Autodesk Inventor part; units mm, degrees
ref_plane "YZ Plane" through (0, 0, 0) normal (1, 0, 0) x (0, 1, 0)
ref_plane "XZ Plane" through (0, 0, 0) normal (0, 1, 0) x (-1, 0, 0)
ref_plane "XY Plane" through (0, 0, 0) normal (0, 0, 1) x (1, 0, 0)
sketch "Sketch1" plane through (0, 0, 0) normal (0, 0, 1) x (1, 0, 0)
  line L0 (2.2943, 2.9258) -> (2.2943, -105.0242)
  line L1 (2.2943, 2.9258) -> (90.7218, 64.8434)
  line L2 (90.7218, 64.8434) -> (27.6787, -10.2885)
  line L3 (2.2943, -105.0242) -> (27.6787, -10.2885)
  point P0 (0, 0)
  dimension "d0" = 107.95
  dimension "d1" = 107.95
extrude "Extrusion1" add sketch "Sketch1" along normal blind 3.175
sketch "Sketch2" plane through (0, 0, 0) normal (0, 0, -1) x (-1, 0, 0)
  line L0 (-2.2943, 2.9258) -> (-2.2943, -105.0242)
  line L1 (-2.2943, -51.0492) -> (-5.4693, -51.0492)
  line L2 (-5.4693, -51.0492) -> (-5.4693, -12.9492)
  line L3 (-5.4693, -12.9492) -> (-2.2943, -12.9492)
  point P0 (0, 0)
  dimension "d8" = 3.175
  dimension "d9" = 38.1
extrude "Extrusion2" add sketch "Sketch2" along normal blind 79.2734
sketch "Sketch3" plane through (2.2943, -105.0242, 3.175) normal (-1, 0, 0) x (0, 0, 1)
  line L0 (-82.4484, 92.075) -> (-63.3984, 92.075)
  line L1 (-63.3984, 92.075) -> (-63.3984, 73.025)
  line L2 (-63.3984, 73.025) -> (-82.4484, 73.025)
  line L3 (-82.4484, 73.025) -> (-82.4484, 92.075)
  point P0 (-3.175, 105.0242)
  dimension "d12" = 19.05
  dimension "d13" = 19.05
hole "Hole1" at (2.2943, -31.9992, -60.2234) direction (1, 0, 0) diameter 8.3312 end through all
properties part number "Left Hip"
Check sheet for the modelled part. Datum: model origin and axes. Units: mm. A direction names the side the tool comes from. Coordinates: 2 decimals unless noted, no trailing zeros. Write each loop counter-clockwise with the first axis right and the second up, starting at its lowest first coordinate (ties: lowest second). Pieces come first, ordered by that corner, then holes. Notation, with made-up numbers: (25.25, -4.75) -> (66.25, -4.75) arc R29 ccw to (66.25, 29.25) -> close; hole circle Ø11 at (-15.5, 34). An arc over 180 degrees is marked (long way). Use a Markdown table: item, result.
1. Sectioned sample at D-D (x = 30). Enter the section's corners in (y, z) (3 decimals).
Reported:
| item | result |
|---|---|
| outline | (-7.522, 0) -> (22.326, 0) -> (22.326, 3.175) -> (-7.522, 3.175) -> close |
2. Sectioned sample at A-A (z = -62). Enter the section's corners in (x, y).
Reported:
| item | result |
|---|---|
| outline | (2.29, -51.05) -> (5.47, -51.05) -> (5.47, -35.77) -> (2.29, -35.77) -> close; (2.29, -28.23) -> (5.47, -28.23) -> (5.47, -12.95) -> (2.29, -12.95) -> close |
3. Go/stop test with flat-tipped pins: pin 1 Ø1 at (x, z) = (3.5, -22.5) entering from -Y; pin 2 Ø3.5 at (x, z) = (3.5, -46) entering from +Y. Record where each tip stops, or that it passes through.
Reported:
| item | result |
|---|---|
| pin 1 | stops at y = -51.05 |
| pin 2 | stops at y = -12.95 |
4. Scan lines: line 1 along Z through (x, y) = (33, 9) (3 decimals); line 2 along X through (y, z) = (-27, -27.5). Record each from-to range of solid material in increasing order.
Reported:
| item | result |
|---|---|
| line 1 | z = 0 to 3.175 |
| line 2 | x = 2.29 to 5.47 |
5. Release check for a two-part mould opening along Z. For faces 6 (the flat face through (4, -32, -79.273)), 7 (the flat face through (2.294, -38, -39)), 8 (the cylindrical face through (3.904, -29.464, -63.529)) record: pulls with the +Z half, pulls with the -Z half, needs draft (parallel to the pull), parting line crosses it, or undercut.
Reported:
| item | result |
|---|---|
| face 6 | pulls with the -Z half |
| face 7 | needs draft |
| face 8 | undercut |
6. Tool access check on faces 1 (the flat face through (27, -7, 3.175)), 2 (the flat face through (4, -12.949, -39)), 3 (the flat face through (5.469, -32, -39)), 4 (the flat face through (4, -51.049, -39)), 5 (the flat face through (14.81, -58.32, 1.57)). Record the directions out of +Z, -Z, +X, -X, +Y, -Y that give a thin tool (end or side, any length) a straight path to the whole face; none if there is none.
Reported:
| item | result |
|---|---|
| face 1 | +Z, +X, -X, +Y, -Y |
| face 2 | -Z, +X, -X, +Y |
| face 3 | -Z, +X, +Y, -Y |
| face 4 | -Z, +X, -X, -Y |
| face 5 | +Z, -Z, +X, -Y |
7. Sectioned sample at C-C (z = -42). Enter the section's corners in (x, y), plus the area to 3 significant figures.
Reported:
| item | result |
|---|---|
| outline | (2.29, -51.05) -> (5.47, -51.05) -> (5.47, -12.95) -> (2.29, -12.95) -> close |
| area | 121 mm2 |
8. Sectioned sample at B-B (y = -47). Enter the section's corners in (x, z) (3 decimals), plus the area to 3 significant figures.
Reported:
| item | result |
|---|---|
| outline | (2.294, -79.273) -> (5.469, -79.273) -> (5.469, 0) -> (17.842, 0) -> (17.842, 3.175) -> (2.294, 3.175) -> close |
| area | 301 mm2 |
